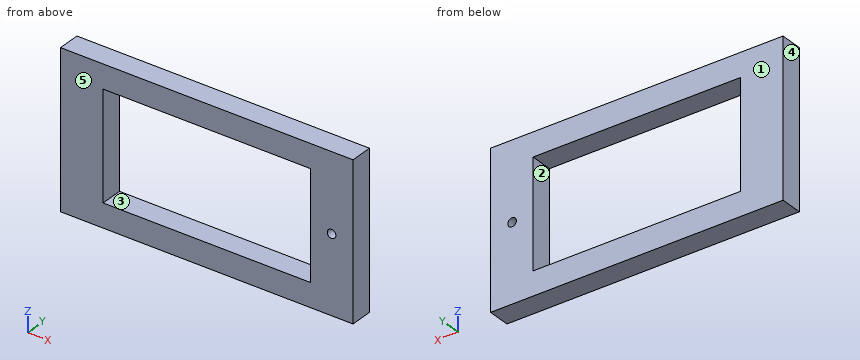
from build123d import *

# Parameters (mm, degrees)
SKETCH_W        = 34.16
SKETCH_H        = 18.11
PAD_DEPTH       = 2.6
SKETCH002_W     = 24.23
SKETCH002_H     = 12.56
POCKET_DEPTH    = 2.6
SKETCH003_R     = 0.5
SKETCH003_W     = 2.01
SKETCH003_H     = 3.5
POCKET001_DEPTH = 5


with BuildPart() as part:
    # Sketch → Pad (new body)
    with BuildSketch(Plane.XZ):
        with Locations((17.08, 9.055)):
            Rectangle(SKETCH_W, SKETCH_H)
    extrude(amount=PAD_DEPTH)

    # Sketch002 (on Face6 of Pad) → Pocket (cut)
    with BuildSketch(Plane.XZ.offset(2.6)):
        with Locations((17.08, 9.055)):
            Rectangle(SKETCH002_W, SKETCH002_H)
    extrude(amount=-POCKET_DEPTH, mode=Mode.SUBTRACT)

    # Sketch003 (on Face4 of Pocket) → Pocket001 (cut)
    with BuildSketch(Plane(origin=(0, 0, 0), x_dir=(1, 0, 0), z_dir=(0, 1, 0))):
        with Locations((31.645, -9.028)):
            Circle(SKETCH003_R)
        with Locations((27.953742, -8.544061)):
            Rectangle(SKETCH003_W, SKETCH003_H)
    extrude(amount=-POCKET001_DEPTH, mode=Mode.SUBTRACT)


solid = part.part
Check sheet for the modelled part. Datum: model origin and axes. Units: mm. Face numbers are marked on the shaded views. A direction names the side the tool comes from. Round coordinates to 2 decimals unless told otherwise and drop trailing zeros. Loops run counter-clockwise (first coordinate to the right, second up) from the corner with the lowest first, then second, coordinate; pieces in that order, holes last. Notation, with made-up numbers: M 57.5,1.25 L 96.5,1.25 A22 cw 96.5,11.25 Z; hole C 45,74 d11. An arc over 180 degrees is marked long. One line per question, with ' | ' between items. Start each with the question number.
Item 1: Scan lines: probe 1 along X at (y, z) = (-1.65, 7) (3 decimals); probe 2 along Z at (x, y) = (14, -0.3) (3 decimals); probe 3 along X at (y, z) = (-1.45, 9.25) (3 decimals). Record each from-to range of solid material in increasing order.
Item 2: Section check A-A (x = 5.5). Record the boundary of the cut face in (y, z) (3 decimals), and give its area (3 significant figures).
Item 3: Section check C-C (y = -1.5). Record the boundary of the cut face in (x, z) (3 decimals), and give its area (3 significant figures).
Item 4: Section check B-B (z = 6.5). Record the boundary of the cut face in (x, y) (3 decimals).
Item 5: Set-up check for the marked faces 1 and 2: record each of +Z, -Z, +X, -X, +Y, -Y from which the full face is reachable in a straight line by a thin tool's end or side.
Item 6: Release check for a two-part mould opening along X. For the marked faces 3, 4 and 5 record: released by +X, released by -X, zero draft, split by the parting line, or undercut.
Worked out:
1) probe 1: 0 to 4.965, 29.195 to 34.16 | probe 2: 0 to 2.775, 15.335 to 18.11 | probe 3: 0 to 4.965, 29.195 to 31.197, 32.093 to 34.16
2) outline: M -2.6,0 L 0,0 L 0,2.775 L -2.6,2.775 Z; M -2.6,15.335 L 0,15.335 L 0,18.11 L -2.6,18.11 Z | area: 14.4 mm^2
3) outline: M 0,0 L 34.16,0 L 34.16,18.11 L 0,18.11 Z; hole M 4.965,2.775 L 29.195,2.775 L 29.195,15.335 L 4.965,15.335 Z; hole C 31.645,9.028 d1 | area: 314 mm^2
4) outline: M 0,-2.6 L 4.965,-2.6 L 4.965,0 L 0,0 Z; M 29.195,-2.6 L 34.16,-2.6 L 34.16,0 L 29.195,0 Z
5) face 1: +Z, -Z, +X, -X, +Y | face 2: +Y, -Y
6) face 3: undercut | face 4: released by -X | face 5: zero draft
